Autodesk Inventor part; units mm, degrees
ref_plane "YZ Plane" through (0, 0, 0) normal (1, 0, 0) x (0, 1, 0)
ref_plane "XZ Plane" through (0, 0, 0) normal (0, 1, 0) x (-1, 0, 0)
ref_plane "XY Plane" through (0, 0, 0) normal (0, 0, 1) x (1, 0, 0)
sketch "Sketch1" plane through (0, 0, 0) normal (0, 0, 1) x (1, 0, 0)
  line L0 (-2.54, -8.19) -> (2.54, -8.19)
  line L1 (2.54, -8.19) -> (2.54, 8.19)
  line L2 (-2.54, 8.19) -> (-2.54, -8.19)
  line L3 (-2.54, -8.19) -> (2.54, 8.19) construction
  line L4 (2.54, -8.19) -> (-2.54, 8.19) construction
  circle A0 centre (0, 16.6545) radius 2.5 construction
  circle A1 centre (0, 16.6545) radius 5
  arc A2 (6.8029, 15.0051) -> (-6.8044, 15.0114) centre (0, 16.6545) ccw
  line L5 (-2.54, 8.19) -> (-2.54, 10.2591)
  line L6 (2.54, 8.19) -> (2.54, 10.2869)
  line L7 (0, 0) -> (0, 10.7842) construction
  line L8 (-2.54, 10.2591) -> (-3.9944, 10.2511)
  line L9 (2.54, 10.2869) -> (3.9944, 10.2948)
  line L10 (-3.9944, 10.2511) -> (-4.1214, 3.9003)
  line L11 (3.9944, 10.2948) -> (4.1214, 3.9454)
  line L12 (-4.1214, 3.9003) -> (-6.8044, 15.0114)
  line L13 (4.1214, 3.9454) -> (6.8029, 15.0051)
  line L14 (0, 0) -> (0, 22.9511) construction
  point P0 (-3.2672, 10.2551)
  dimension "d2" = 5
  dimension "d3" = 10
  dimension "d4" = 14
  dimension "d8" = 1.5815
  dimension "d9" = 1.5815
  dimension "d10" = 6.35
  dimension "d11" = 6.35
  dimension "d18" = 1.4545
  dimension "d19" = 1.4545
  dimension "d31" = 2.54
  dimension "d32" = 2.54
  dimension "d33" = 0
extrude "Plate1" add sketch "Sketch1" along normal blind 3.175
sketch "Sketch2" plane through (0, 0, 0) normal (0, 0, -1) x (-1, 0, 0)
  circle A0 centre (0, 16.6545) radius 5
  line L0 (-3.9944, 10.2948) -> (-4.1214, 3.9454)
  line L1 (-2.54, 10.2869) -> (-3.9944, 10.2948)
  line L2 (-2.54, -8.19) -> (-2.54, 10.2869)
  line L3 (2.54, -8.19) -> (-2.54, -8.19)
  line L4 (2.54, 10.2591) -> (2.54, -8.19)
  line L5 (3.9944, 10.2511) -> (2.54, 10.2591)
  line L6 (4.1214, 3.9003) -> (3.9944, 10.2511)
  line L7 (6.8044, 15.0114) -> (4.1214, 3.9003)
  arc A1 (6.8044, 15.0114) -> (-6.8029, 15.0051) centre (0, 16.6545) ccw
  line L8 (-4.1214, 3.9454) -> (-6.8029, 15.0051)
  line L9 (-1.5875, -17.19) -> (1.5875, -17.19)
  line L10 (1.5875, -17.19) -> (1.5875, 0.81)
  line L11 (1.5875, 0.81) -> (-1.5875, 0.81)
  line L12 (-1.5875, 0.81) -> (-1.5875, -17.19)
  line L13 (-1.5875, -17.19) -> (1.5875, 0.81) construction
  line L14 (1.5875, -17.19) -> (-1.5875, 0.81) construction
  point P0 (0, 0)
  point P1 (0, -8.19)
  dimension "d14" = 3.175
extrude "Extrusion1" cut sketch "Sketch2" against normal blind 25.4 contours L12 L11 L10 L3 | L3 L10 L9 L12
sketch "Sketch3" plane through (0, 0, 3.175) normal (0, 0, 1) x (1, 0, 0)
  circle A0 centre (-37.757, 0) radius 3
  line L0 (-39.3445, -2.5456) -> (-36.1695, -2.5456)
  line L1 (-36.1695, -2.5456) -> (-36.1695, 2.5456)
  line L2 (-36.1695, 2.5456) -> (-39.3445, 2.5456)
  line L3 (-39.3445, 2.5456) -> (-39.3445, -2.5456)
  line L4 (-39.3445, -2.5456) -> (-36.1695, 2.5456) construction
  line L5 (-36.1695, -2.5456) -> (-39.3445, 2.5456) construction
  circle A1 centre (-37.757, 0) radius 4
  point P0 (0, 0)
  point P1 (-37.757, 3)
  point P2 (-37.757, 4)
  dimension "d35" = 8
  dimension "d28" = 6
  dimension "d29" = 3.175
  dimension "d30" = 5.0911
  dimension "d34" = 0.4545
  dimension "d36" = 1.4545
fillet "Fillet4" radius 0.381 6 edges at (-4.1214, 3.9003, 1.5875) (4.1214, 3.9454, 1.5875) (-2.54, -8.19, 1.5875) (-1.5875, -8.19, 1.5875) (1.5875, -8.19, 1.5875) (2.54, -8.19, 1.5875)
ref_plane "Work Plane1" through (0, 10.2591, 0) normal (-1, 0, 0) x (0, 0, 1)
ref_plane "Work Plane2" through (0, 0, 1.5875) normal (0, 0, 1) x (1, 0, 0)
chamfer "Chamfer3" distance 0.127 distance2 3.175 1 edges at (-2.54, 10.2591, 1.5875) measured on face at (-3.5096, 10.2538, 1.0583)
chamfer "Chamfer4" distance 3.175 distance2 0.127 1 edges at (2.54, 10.2869, 1.5875) measured on face at (2.54, -1.7771, 1.0583)
equation "\"d18\" = d36"
equation "\"d19\" = d36"
equation "\"BendRadius\" = Thickness"
equation "\"BendReliefWidth\" = Thickness"
equation "\"BendReliefDepth\" = 0.5 * Thickness"
equation "\"CornerReliefSize\" = 4 * Thickness"
equation "\"MinimumRemnant\" = 2 * Thickness"
equation "\"TransitionRadius\" = BendRadius"
equation "\"JacobiRadiusSize\" = BendRadius"
equation "\"GapSize\" = Thickness"
equation "\"d12\" = BendRadius"
properties part number "8mm OD 6mm ID Rod End125"
Read the model definition and answer for the solid it produces. Units are mm, in the model's axes. A direction names the side the tool comes from. Coordinates: 2 decimals unless noted, no trailing zeros. Write each loop counter-clockwise with the first axis right and the second up, starting at its lowest first coordinate (ties: lowest second). Pieces come first, ordered by that corner, then holes. Notation, with made-up numbers: (-22, 13) - (16, 13) arc R29 cw to (16, 35) - close; hole circle Ø9 at (23, 23.25). An arc over 180 degrees is marked (long way). Answer as a JSON object with one key per item and string values. Group by question number.
1. A cutting plane is placed at B-B (y = 18.5). Determine the outline of the cut face in (x, z) (3 decimals), plus the area to 3 significant figures.
2. A cutting plane is placed at A-A (x = 0). Determine the outline of the cut face in (y, z) (1 decimal), plus the area to 3 significant figures.
3. A cutting plane is placed at D-D (y = 6). Determine the outline of the cut face in (x, z) (3 decimals), plus the area to 3 significant figures.
4. The mould has two halves that part along Y. Classify faces 1 (the flat face through (0, 11, 0)), 2 (the cylindrical face through (-0.651, 11.697, 1.565)), 3 (the flat face through (-2.6, 8.6, 1.6)): +Y half, -Y half, draft (parallel to the pull), parting line (faces both ways), or undercut.
5. Which of the six approach directions +Z, -Z, +X, -X, +Y, -Y give full straight-line access (tool end or side, diameter ignored) to faces 4 (the cylindrical face through (-0.174, 23.652, 1.565)), 5 (the flat face through (0, 0.81, 2))?
6. Each of these flat-tipped pins is pushed along its axis until it touches: P1, Ø1.6, axis at x = 0.5, z = 2, coming from the -Y side; P2, Ø1.6, axis at y = -2.5, z = 2.5, coming from the +X side; P3, Ø1.6, axis at y = -3.5, z = 1, coming from the -X side; P4, Ø8, axis at x = 4.5, y = 9.5, coming from the -Z side. Where does it stop, or does it pass through?
7. A cutting plane is placed at C-C (z = 2.4). Determine the outline of the cut face in (x, y), plus the area to 3 significant figures.
8. Consider L1, parallel to Y at x = 0, z = 1.2; L2, parallel to X at y = -4.5, z = 2; L3, parallel to X at y = 7.5, z = 0.3. Determine where each line is inside the solid, lowest interval first. Write a range as [from, to].
Worked out:
{
 "1": {"outline": "(-6.752, 0) - (-4.647, 0) - (-4.647, 3.175) - (-6.752, 3.175) - close; (4.647, 0) - (6.752, 0) - (6.752, 3.175) - (4.647, 3.175) - close", "area": "13.4 mm²"},
 "2": {"outline": "(0.8, 0) - (11.7, 0) - (11.7, 3.2) - (0.8, 3.2) - close; (21.7, 0) - (23.7, 0) - (23.7, 3.2) - (21.7, 3.2) - close", "area": "40.8 mm²"},
 "3": {"outline": "(-2.54, 0) - (2.54, 0) - (2.54, 3.175) - (-2.54, 3.175) - close", "area": "16.1 mm²"},
 "4": {"face 1": "draft", "face 2": "undercut", "face 3": "-Y half"},
 "5": {"face 4": "+Z, -Z", "face 5": "+Z, -Z, -Y"},
 "6": {"P1": "stops at y = 0.81", "P2": "stops at x = 2.54", "P3": "stops at x = -2.54", "P4": "stops at z = 0"},
 "7": {"outline": "(-6.8, 15.01) - (-4.81, 6.77) arc R0.38 ccw to (-4.06, 6.85) - (-3.99, 10.25) - (-2.67, 10.26) - (-2.54, 7.08) - (-2.54, -7.81) arc R0.38 ccw to (-2.16, -8.19) - (-1.97, -8.19) arc R0.38 ccw to (-1.59, -7.81) - (-1.59, 0.81) - (1.59, 0.81) - (1.59, -7.81) arc R0.38 ccw to (1.97, -8.19) - (2.16, -8.19) arc R0.38 ccw to (2.54, -7.81) - (2.54, 7.11) - (2.67, 10.29) - (3.99, 10.29) - (4.06, 6.88) arc R0.38 ccw to (4.81, 6.8) - (6.8, 15.01) arc R7 ccw (long way) to start; hole circle Ø10 at (0, 16.65)", "area": "155 mm²"},
 "8": {"L1": "y = [0.81, 11.65], [21.65, 23.65]", "L2": "x = [-2.54, -1.59], [1.59, 2.54]", "L3": "x = [-4.99, -4.05], [-2.56, 2.56], [4.05, 4.98]"}
}
